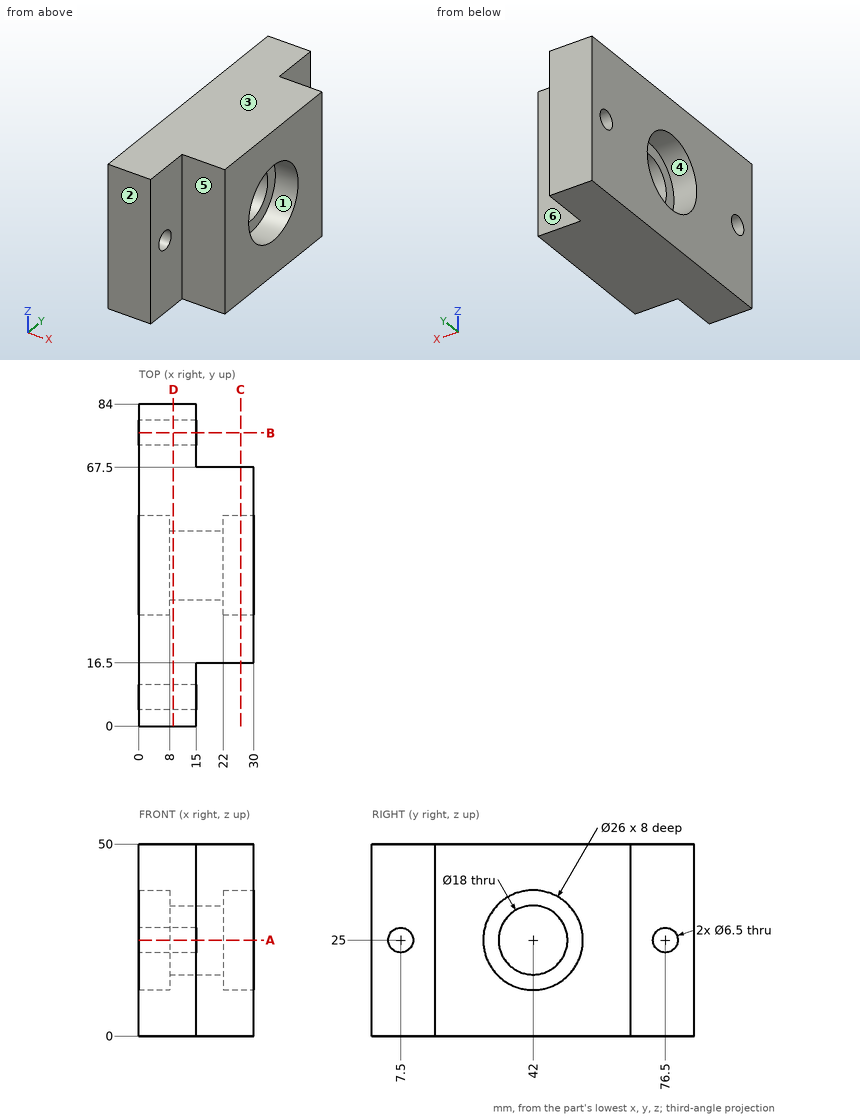
Answer from the drawing. Dimensions are ordinates in mm from the lowest x, y and z of the part. A direction names the side the tool comes from. Round coordinates to 2 decimals unless told otherwise and drop trailing zeros. Write each loop counter-clockwise with the first axis right and the second up, starting at its lowest first coordinate (ties: lowest second). Pieces come first, ordered by that corner, then holes. Notation, with made-up numbers: (10.25, -34.75) -> (39.25, -34.75) arc R19 cw to (39.25, -5.75) -> close; hole circle Ø11 at (-26.5, 11.5). An arc over 180 degrees is marked (long way). Answer in a Markdown table with one row per item. Add a question column.
1) Find section D-D, the plane x = 9. Determine the outline of the cut face in (y, z), and give its area (3 significant figures).
2) Which of the six approach directions +Z, -Z, +X, -X, +Y, -Y give full straight-line access (tool end or side, diameter ignored) to the marked faces 4, 5 and 6?
3) Given P1, Ø8, axis at y = 41, z = 30.5, coming from the +X side; P2, Ø7.5, axis at x = 26, z = 36, coming from the -Y side; P3, Ø2, axis at x = 4.5, y = 73, coming from the -Z side; P4, Ø21, axis at y = 42, z = 25, coming from the -X side, each flat-ended and moving along its own axis, determine where each tip first touches the part or whether it passes through.
4) Find section C-C, the plane x = 26.5. Determine the outline of the cut face in (y, z), and give its area (3 significant figures).
5) Consider line 1 (Y direction, x = 5.75, z = 25); line 2 (Y direction, x = 23.25, z = 25); line 3 (Z direction, x = 25.5, y = 42). Determine where each line is inside the solid, lowest interval first.
6) Find section B-B, the plane y = 76.5. Determine the outline of the cut face in (x, z).
7) Determine the mould class of the marked faces 1, 2 and 3 for opening direction Z: pulls with the +Z half, pulls with the -Z half, needs draft (parallel to the pull), parting line crosses it, or undercut.
8) Find section A-A, the plane z = 25. Determine the outline of the cut face in (x, y), and give its area (3 significant figures).
Findings below:
| question | item | result |
|---|---|---|
| 1 | outline | (0, 0) -> (84, 0) -> (84, 50) -> (0, 50) -> close; hole circle Ø6.5 at (7.5, 25); hole circle Ø18 at (42, 25); hole circle Ø6.5 at (76.5, 25) |
| 1 | area | 3,880 mm² |
| 2 | face 4 | -X |
| 2 | face 5 | +Z, -Z, +X, -Y |
| 2 | face 6 | +Z, -Z, +X, +Y |
| 3 | P1 | x = 22 |
| 3 | P2 | y = 16.5 |
| 3 | P3 | z = 0 |
| 3 | P4 | x = 8 |
| 4 | outline | (16.5, 0) -> (67.5, 0) -> (67.5, 50) -> (16.5, 50) -> close; hole circle Ø26 at (42, 25) |
| 4 | area | 2,020 mm² |
| 5 | line 1 | 0 to 4.25, 10.75 to 29, 55 to 73.25, 79.75 to 84 |
| 5 | line 2 | 16.5 to 29, 55 to 67.5 |
| 5 | line 3 | 0 to 12, 38 to 50 |
| 6 | outline | (0, 0) -> (15, 0) -> (15, 21.75) -> (0, 21.75) -> close; (0, 28.25) -> (15, 28.25) -> (15, 50) -> (0, 50) -> close |
| 7 | face 1 | undercut |
| 7 | face 2 | needs draft |
| 7 | face 3 | pulls with the +Z half |
| 8 | outline | (0, 0) -> (15, 0) -> (15, 4.25) -> (0, 4.25) -> close; (0, 10.75) -> (15, 10.75) -> (15, 16.5) -> (30, 16.5) -> (30, 29) -> (22, 29) -> (22, 33) -> (8, 33) -> (8, 29) -> (0, 29) -> close; (0, 55) -> (8, 55) -> (8, 51) -> (22, 51) -> (22, 55) -> (30, 55) -> (30, 67.5) -> (15, 67.5) -> (15, 73.25) -> (0, 73.25) -> close; (0, 79.75) -> (15, 79.75) -> (15, 84) -> (0, 84) -> close |
| 8 | area | 1,160 mm² |
